Could you check a few things on this model? Use its own coordinates, in mm. A direction names the side the tool comes from. Coordinates: 2 decimals unless noted, no trailing zeros. Write each loop counter-clockwise with the first axis right and the second up, starting at its lowest first coordinate (ties: lowest second). Pieces come first, ordered by that corner, then holes.
Item 1: For P1, Ø0.5, axis at y = -2, z = 0.5, coming from the -X side; P2, Ø0.5, axis at y = 2, z = 0.5, coming from the +X side, each with a flat end and sliding along its axis, tell me the tip position at first contact or that it passes through.
Item 2: I want a section at B-B on x = -0.25. Please give me the cut outline in (y, z), then the cut area to 3 significant figures.
Item 3: Thinking about a two-plate mould opening in Y: for faces 1 (the cylindrical face through (3.233, -1.341, 0.493)), 2 (the flat face through (0, -1, 0)), 3 (the cylindrical face through (0.567, 1.389, 0.493)), which applies, +Y half, -Y half, draft (parallel to the pull), parting line (faces both ways), or undercut?
Item 4: I want a section at A-A on x = 2.5. Please give me the cut outline in (y, z), then the cut area to 3 significant figures.
Item 5: Which directions (+Z, -Z, +X, -X, +Y, -Y) give clear straight access to the entire face, cutting with the end or side of a thin tool? Please do faces 4 (the cylindrical face through (-2.4, 1, 0.5)), 5 (the flat face through (0, -1, 1)).
Item 6: If I drill on probe 1 along Y at (x, z) = (0, 0.25); probe 2 along Y at (x, z) = (-0.25, 0.25); probe 3 along X at (y, z) = (-1.25, 0.2), over which ranges is the centre line in solid material (lowest first)?
Item 7: I want a section at D-D on y = 1.25. Please give me the cut outline in (x, z).
Item 8: I want a section at C-C on z = 0.25. Please give me the cut outline in (x, y).
from build123d import *

# Parameters (mm, degrees)
SKETCH2_R           = 3.5
BOSS_EXTRUDE1_DEPTH = 1
SKETCH4_R           = 0.4
CUT_EXTRUDE2_DEPTH  = 6.049752469
CUT_EXTRUDE3_START  = -1
CUT_EXTRUDE3_DEPTH  = 1
CIRPATTERN1_COUNT   = 4


# Read off the part's stored shape, not the designer's step: Cut-Extrude3
with BuildPart() as part:
    # Sketch2 → Boss-Extrude1 (new body)
    with BuildSketch(Plane.XY):
        Circle(SKETCH2_R)
    extrude(amount=BOSS_EXTRUDE1_DEPTH)

    # Sketch4 → Cut-Extrude2 (cut, through all)
    with BuildSketch(Plane.XY.offset(1)):
        Circle(SKETCH4_R)
    extrude(amount=-CUT_EXTRUDE2_DEPTH, mode=Mode.SUBTRACT)

    # Cut-Extrude3 outline → Cut-Extrude3 (cut)
    with BuildSketch(Plane.XY.offset(1).offset(CUT_EXTRUDE3_START)):
        with BuildLine():
            ThreePointArc((-0.05, -1.499166435), (-0.574025148, -1.385819299), (-1.024715413, -1.095426092))
            Line((-1.024715413, -1.095426092), (-1.802782305, -1.873492984))
            ThreePointArc((-1.802782305, -1.873492984), (-0.994976924, -2.402086785), (-0.05, -2.599519186))
            Line((-0.05, -2.599519186), (-0.05, -1.499166435))
        make_face()
    cut_extrude3 = extrude(amount=CUT_EXTRUDE3_DEPTH, mode=Mode.SUBTRACT)

    # CirPattern1: Cut-Extrude3 ×4 about axis
    cirpattern1_axis = Axis((0, 0, 0), (0, 0, 1))
    for i in range(1, CIRPATTERN1_COUNT):
        add(cut_extrude3.rotate(cirpattern1_axis, i * 360 / CIRPATTERN1_COUNT), mode=Mode.SUBTRACT)


solid = part.part
Response values:
1. P1: stops at x = -3.03
1. P2: stops at x = 3.03
2. outline: (-3.49, 0) - (-2.59, 0) - (-2.59, 1) - (-3.49, 1) - close; (-1.48, 0) - (-0.31, 0) - (-0.31, 1) - (-1.48, 1) - close; (0.31, 0) - (3.49, 0) - (3.49, 1) - (0.31, 1) - close
2. area: 5.25 mm2
3. face 1: parting line
3. face 2: draft
3. face 3: undercut
4. outline: (-2.45, 0) - (-0.71, 0) - (-0.71, 1) - (-2.45, 1) - close; (-0.05, 0) - (2.45, 0) - (2.45, 1) - (-0.05, 1) - close
4. area: 4.23 mm2
5. face 4: +Z, -Z
5. face 5: +Z, +X, -X, +Y, -Y
6. probe 1: y = -3.5 to -0.4, 0.4 to 3.5
6. probe 2: y = -3.49 to -2.59, -1.48 to -0.31, 0.31 to 3.49
6. probe 3: x = -3.27 to -1.18, -0.83 to 1.32, 2.28 to 3.27
7. outline: (-3.27, 0) - (-2.28, 0) - (-2.28, 1) - (-3.27, 1) - close; (-1.32, 0) - (0.83, 0) - (0.83, 1) - (-1.32, 1) - close; (1.18, 0) - (3.27, 0) - (3.27, 1) - (1.18, 1) - close
8. outline: circle Ø7 at (0, 0); hole (-2.6, 0.05) - (-1.5, 0.05) arc R1.5 cw to (-1.1, 1.02) - (-1.87, 1.8) arc R2.6 ccw to start; hole (-1.8, -1.87) arc R2.6 ccw to (-0.05, -2.6) - (-0.05, -1.5) arc R1.5 cw to (-1.02, -1.1) - close; hole circle Ø0.8 at (0, 0); hole (0.05, 1.5) arc R1.5 cw to (1.02, 1.1) - (1.8, 1.87) arc R2.6 ccw to (0.05, 2.6) - close; hole (1.1, -1.02) - (1.87, -1.8) arc R2.6 ccw to (2.6, -0.05) - (1.5, -0.05) arc R1.5 cw to start
